```python
from build123d import *

# Parameters (mm, degrees)
SKETCH1_R             = 3.475
BOSS_EXTRUDE1_DEPTH   = 42
CHAMFER1_SIZE         = 0.2
CHAMFER1_SIZE2        = 0.346410162
CHAMFER1_PART_2_SIZE  = 0.2
CHAMFER1_PART_2_SIZE2 = 0.346410162


with BuildPart() as part:
    # Sketch1 → Boss-Extrude1 (new body, symmetric)
    with BuildSketch(Plane.XY):
        Circle(SKETCH1_R)
    extrude(amount=BOSS_EXTRUDE1_DEPTH, both=True)

    # Chamfer1
    chamfer1_edges = [part.edges().sort_by_distance(p)[0] for p in [
        (-3.475, 0, -42),
    ]]
    chamfer1_side = [part.faces().sort_by_distance(p)[0] for p in [
        (0, 0, -42),
    ]]
    chamfer(chamfer1_edges, length=CHAMFER1_SIZE, length2=CHAMFER1_SIZE2, reference=chamfer1_side[0])

    # Chamfer1 part 2
    chamfer1_part_2_edges = [part.edges().sort_by_distance(p)[0] for p in [
        (-3.475, 0, 42),
    ]]
    chamfer1_part_2_side = [part.faces().sort_by_distance(p)[0] for p in [
        (-3.475, 0, 0),
    ]]
    chamfer(chamfer1_part_2_edges, length=CHAMFER1_PART_2_SIZE, length2=CHAMFER1_PART_2_SIZE2, reference=chamfer1_part_2_side[0])


solid = part.part
```
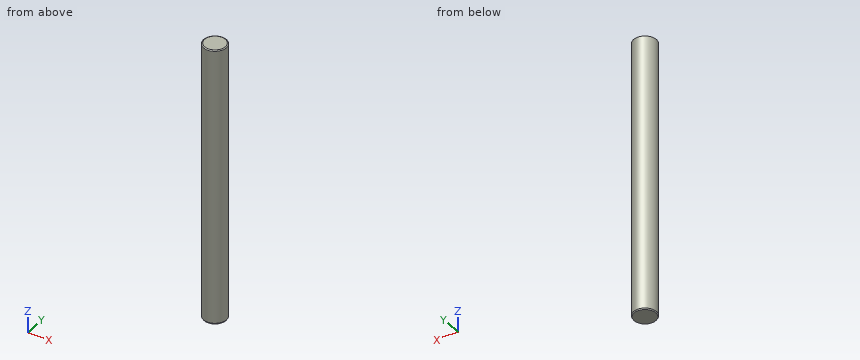
Source: CAD feature listing. Evaluate the final solid. Frame: model axes, mm. Coordinates: 2 decimals unless noted, no trailing zeros. Loops run counter-clockwise (first coordinate to the right, second up) from the corner with the lowest first, then second, coordinate; pieces in that order, holes last. Notation, with made-up numbers: M 52.25,68 L 101.25,68 A23 ccw 101.25,95 Z; hole C -29,43.25 d11. An arc over 180 degrees is marked long. Use a Markdown table: item, result. Add a question column.
Q1. Material intervals for L1, parallel to X at y = 0.25, z = 38.5; L2, parallel to Y at x = -0.5, z = -7.5, sorted ascending.
Q2. Section query A-A, the plane z = 14. Return loops of the section in (x, y) (3 decimals), and give its area (3 significant figures).
Q3. First-contact query: pin 1 (1 mm diameter, centred on x = 0.5, z = 33, fed in from +Y) (3 decimals); pin 2 (1.5 mm diameter, centred on y = 2, z = -22, fed in from -X); pin 3 (1.5 mm diameter, centred on x = -2.5, z = -6, fed in from +Y). Flat tips, straight axial feed; report the tip coordinate or a pass-through.
Result:
| question | item | result |
|---|---|---|
| 1 | L1 | x = -3.47 to 3.47 |
| 1 | L2 | y = -3.44 to 3.44 |
| 2 | outline | C 0,0 d6.95 |
| 2 | area | 37.9 mm2 |
| 3 | pin 1 | stops at y = 3.475 |
| 3 | pin 2 | stops at x = -3.24 |
| 3 | pin 3 | stops at y = 3 |
